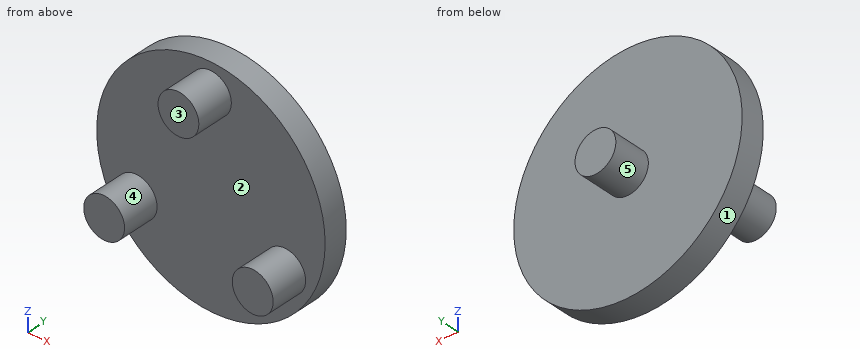
from build123d import *

# Parameters (mm, degrees)
F0_R     = 6.15
F1_DEPTH = 1.3
F2_R     = 1.1
F3_DEPTH = 2
F4_R     = 1.1
F5_DEPTH = 2


with BuildPart() as f1:
    # F0 (on Front) → F1 (new body)
    with BuildSketch(Plane.XZ):
        Circle(F0_R)
    extrude(amount=F1_DEPTH)

    # F2 (on face) → F3 (join)
    with BuildSketch(Plane.XZ.offset(1.3)):
        with Locations((0, 4.62)):
            Circle(F2_R)
        with Locations((-4.0010373655, -2.31)):
            Circle(F2_R)
        with Locations((4.0010373655, -2.31)):
            Circle(F2_R)
    extrude(amount=F3_DEPTH)

    # F4 (on face) → F5 (join)
    with BuildSketch(Plane(origin=(0, 0, 0), x_dir=(-1, 0, 0), z_dir=(0, 1, 0))):
        Circle(F4_R)
    extrude(amount=F5_DEPTH)


solid = f1.part
Read the model definition and answer for the solid it produces. Units are mm, in the model's axes. Face numbers are marked on the shaded views. A direction names the side the tool comes from. Give positions to 0.01 mm unless a question says otherwise; leave off trailing zeros. Loops run counter-clockwise (first coordinate to the right, second up) from the corner with the lowest first, then second, coordinate; pieces in that order, holes last. Notation, with made-up numbers: (-25.75, 74.25) - (32.25, 74.25) arc R13 cw to (32.25, 79.25) - close; hole circle Ø1 at (31.5, 68). An arc over 180 degrees is marked (long way). Answer as CSV lines item,"result". Start each with the question number.
1) Each of these flat-tipped pins is pushed along its axis until it touches: pin 1 Ø1.5 at (x, z) = (-4, 3.5) entering from +Y; pin 2 Ø1 at (x, z) = (0, -0.5) entering from -Y; pin 3 Ø1.5 at (x, y) = (1.5, -1) entering from +Z. Where does it stop, or does it pass through?
2) Find section D-D (y = 1.45). Write down the section's boundary in (x, z), then the cut area to 3 significant figures.
3) Find section C-C (x = -4.25). Write down the section's boundary in (y, z).
4) Straight lines are drawn through the part: L1, parallel to Y at x = 4.5, z = 3.25; L2, parallel to Y at x = -4, z = -3; L3, parallel to X at y = -1.2, z = 0.5. For each, find the intervals that lie inside material, in ascending order. Write a range as from..to.
5) Determine the mould class of the marked faces 3, 4 and 5 for opening direction X: released by +X, released by -X, zero draft, split by the parting line, or undercut.
6) Which of the six approach directions +Z, -Z, +X, -X, +Y, -Y give full straight-line access (tool end or side, diameter ignored) to the marked faces 1 and 2?
7) Find section B-B (y = -2.2). Write down the section's boundary in (x, z).
8) Find section A-A (z = 0). Write down the section's boundary in (x, y), then the cut area to 3 significant figures.
Findings below:
1,pin 1,"y = 0"
1,pin 2,"y = -1.3"
1,pin 3,"z = 6.1"
2,outline,"circle Ø2.2 at (0, 0)"
2,area,"3.80 mm^2"
3,outline,"(-3.3, -3.38) - (-1.3, -3.38) - (-1.3, -4.45) - (0, -4.45) - (0, 4.45) - (-1.3, 4.45) - (-1.3, -1.24) - (-3.3, -1.24) - close"
4,L1,"-1.3..0"
4,L2,"-3.3..0"
4,L3,"-6.13..6.13"
5,face 3,"zero draft"
5,face 4,"undercut"
5,face 5,"split by the parting line"
6,face 1,"+Y, -Y"
6,face 2,"-Y"
7,outline,"circle Ø2.2 at (-4, -2.31); circle Ø2.2 at (0, 4.62); circle Ø2.2 at (4, -2.31)"
8,outline,"(-6.15, -1.3) - (6.15, -1.3) - (6.15, 0) - (1.1, 0) - (1.1, 2) - (-1.1, 2) - (-1.1, 0) - (-6.15, 0) - close"
8,area,"20.4 mm^2"
